Verification items for the finished model (mm, model axes). Face numbers are marked on the shaded views. A direction names the side the tool comes from. Round coordinates to 2 decimals unless told otherwise and drop trailing zeros. Order: outer loops, then holes, each group sorted by start corner. A loop starts at its lowest first (then second) coordinate and runs counter-clockwise, first axis right, second up. Notation, with made-up numbers: M 9,-12 L 29,-12 A19 cw 29,18 Z; hole C 9,-19 d11. An arc over 180 degrees is marked long. Return JSON: item names as keys, results as strings. Group by question number.
from build123d import *

# Parameters (mm, degrees)
SKETCH1_R           = 2
BOSS_EXTRUDE1_DEPTH = 20.7
BOSS_EXTRUDE2_DEPTH = 2
CHAMFER1_SIZE       = 0.5
FILLET1_R           = 0.2


with BuildPart() as part:
    # Sketch1 → Boss-Extrude1 (new body)
    with BuildSketch(Plane(origin=(0, 0, 0), x_dir=(1, 0, 0), z_dir=(0, 1, 0))):
        Circle(SKETCH1_R)
    extrude(amount=BOSS_EXTRUDE1_DEPTH)

    # Sketch2 → Boss-Extrude2 (add)
    with BuildSketch(Plane(origin=(0, 20.7, 0), x_dir=(1, 0, 0), z_dir=(0, 1, 0))):
        Polygon((2.5, -1.443375673), (2.5, 1.443375673), (0, 2.886751346), (-2.5, 1.443375673), (-2.5, -1.443375673), (0, -2.886751346), align=None)
    extrude(amount=BOSS_EXTRUDE2_DEPTH)

    # Chamfer1
    chamfer1_edges = [part.edges().sort_by_distance(p)[0] for p in [
        (-2, 0, 0),
    ]]
    chamfer(chamfer1_edges, length=CHAMFER1_SIZE)

    # Fillet1
    fillet1_edges = [part.edges().sort_by_distance(p)[0] for p in [
        (-2, 20.7, 0),
        (1.25, 20.7, 2.165063509),
        (0, 21.7, 2.886751346),
        (2.5, 20.7, 0),
        (2.5, 21.7, 1.443375673),
        (1.25, 20.7, -2.165063509),
        (2.5, 21.7, -1.443375673),
        (-1.25, 20.7, -2.165063509),
        (0, 21.7, -2.886751346),
        (-2.5, 20.7, 0),
        (-2.5, 21.7, -1.443375673),
        (-1.25, 20.7, 2.165063509),
        (-2.5, 21.7, 1.443375673),
        (1.25, 22.7, 2.165063509),
        (2.5, 22.7, 0),
        (1.25, 22.7, -2.165063509),
        (-1.25, 22.7, -2.165063509),
        (-2.5, 22.7, 0),
        (-1.25, 22.7, 2.165063509),
    ]]
    fillet(fillet1_edges, radius=FILLET1_R)


solid = part.part
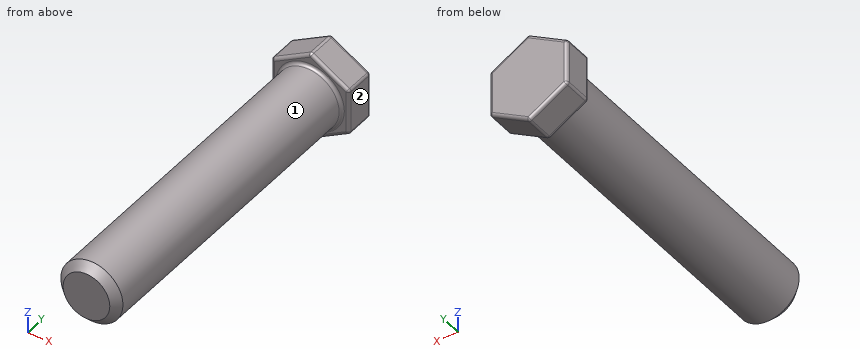
1. Go/stop test with flat-tipped pins: pin 1 (2 mm diameter, centred on y = 7, z = -2, fed in from +X); pin 2 (1.5 mm diameter, centred on y = 19.5, z = -1.5, fed in from -X); pin 3 (2 mm diameter, centred on y = 4.5, z = 1, fed in from +X). Record where each tip stops, or that it passes through.
2. Thickness scan on line 1 along Z through (x, y) = (-0.1, 8.5); line 2 along X through (y, z) = (3.5, -1.5). Record the ranges inside material, lowest first. Write a range as from..to.
3. Cross-section at B-B (y = 10). Enter the section's corners in (x, z), plus the area to 3 significant figures.
4. Access from +Z, -Z, +X, -X, +Y, -Y to the whole of each face (thin tool, end or side, straight path). Record for the marked faces 1 and 2.
5. Cross-section at A-A (z = 0). Enter the section's corners in (x, y), plus the area to 3 significant figures.
Computed:
{
 "1": {"pin 1": "stops at x = 1.73", "pin 2": "stops at x = -1.85", "pin 3": "stops at x = 2"},
 "2": {"line 1": "z = -2..2", "line 2": "x = -1.32..1.32"},
 "3": {"outline": "C 0,0 d4", "area": "12.6 mm²"},
 "4": {"face 1": "-Y", "face 2": "+Z, -Z, +X, +Y, -Y"},
 "5": {"outline": "M -2.5,20.9 A0.2 ccw -2.3,20.7 L -2.2,20.7 A0.2 cw -2,20.5 L -2,0.5 L -1.5,0 L 1.5,0 L 2,0.5 L 2,20.5 A0.2 cw 2.2,20.7 L 2.3,20.7 A0.2 ccw 2.5,20.9 L 2.5,22.5 A0.2 ccw 2.3,22.7 L -2.3,22.7 A0.2 ccw -2.5,22.5 Z", "area": "92.5 mm²"}
}
